Here's how the part is built. I have some questions about the finished solid (model axes, mm). A direction names the side the tool comes from. Give positions to 0.01 mm unless a question says otherwise; leave off trailing zeros. Order: outer loops, then holes, each group sorted by start corner. A loop starts at its lowest first (then second) coordinate and runs counter-clockwise, first axis right, second up.
Autodesk Inventor part; units mm, degrees
ref_plane "YZ Plane" through (0, 0, 0) normal (1, 0, 0) x (0, 1, 0)
ref_plane "XZ Plane" through (0, 0, 0) normal (0, 1, 0) x (-1, 0, 0)
ref_plane "XY Plane" through (0, 0, 0) normal (0, 0, 1) x (1, 0, 0)
sketch "Sketch1" plane through (0, 0, 0) normal (1, 0, 0) x (0, 1, 0)
  circle A0 centre (0, 0) radius 4.25
  circle A1 centre (40, 0) radius 4.25
  circle A2 centre (40, -30) radius 4.25
  circle A3 centre (0, -30) radius 4.25
  circle A4 centre (20, -60) radius 4.25
  line L0 (54.25, 0) -> (54.25, -30)
  line L1 (20, -74.25) -> (54.25, -30)
  line L2 (-14.25, -30) -> (20, -74.25)
  line L3 (-14.25, -30) -> (-14.25, 0)
  line L4 (0, 14.25) -> (54.25, 14.25)
  line L5 (54.25, 14.25) -> (-14.25, 14.25)
  line L6 (-14.25, 14.25) -> (-14.25, 0)
  line L7 (54.25, 14.25) -> (54.25, 0)
  dimension "d6" = 8.5
  dimension "d9" = 8.5
  dimension "d10" = 14.25
  dimension "d11" = 14.25
  dimension "d13" = 14.25
extrude "Extrusion1" add sketch "Sketch1" along normal blind 10
fillet "Fillet1" radius 7 5 edges at (5, 20, -74.25) (5, 54.25, -30) (5, 54.25, 14.25) (5, -14.25, 14.25) (5, -14.25, -30)
sketch "Sketch2" plane through (10, 0, 0) normal (1, 0, 0) x (0, 0, -1)
  circle A0 centre (0, 40) radius 4.25
  line L0 (0, 28) -> (30, 28)
  line L1 (0, 0) -> (0, 12)
  line L2 (0, 12) -> (30, 12)
  circle A1 centre (60, 20) radius 4.25
  arc A2 (45.061, 16.1433) -> (45.061, 23.8567) centre (44, 20) ccw
  line L3 (30, 28) -> (45.061, 23.8567)
  line L4 (30, 12) -> (45.061, 16.1433)
  line L5 (-14.25, 47.25) -> (-14.25, -7.25)
  line L6 (-2.25, 28) -> (0, 28)
  line L7 (-2.25, 28) -> (-2.25, 12)
  line L8 (-2.25, 12) -> (0, 12)
extrude "Extrusion2" cut sketch "Sketch2" against normal up to surface (10 mm away) contours L0 L3 A2 L4 L2 L8 L7 L6
fillet "Fillet2" radius 5 4 edges at (5, 12, -30) (5, 28, -30) (5, 28, 2.25) (5, 12, 2.25)
properties part number "din_motor_connector"
Q1. If we section it at D-D on y = 40: List the corners of the cut face in (x, z) for me.
Filled sheet:
outline: (0, -48.41) - (10, -48.41) - (10, -34.25) - (0, -34.25) - close; (0, -25.75) - (10, -25.75) - (10, -4.25) - (0, -4.25) - close; (0, 4.25) - (10, 4.25) - (10, 14.25) - (0, 14.25) - close
Q2. If we section it at A-A on z = -11.5: List the corners of the cut face in (x, y) for me.
Filled sheet:
outline: (0, -14.25) - (10, -14.25) - (10, 12) - (0, 12) - close; (0, 28) - (10, 28) - (10, 54.25) - (0, 54.25) - close
Q3. If we section it at C-C on y = 20: List the corners of the cut face in (x, z) for me.
Filled sheet:
outline: (0, -69.81) - (10, -69.81) - (10, -64.25) - (0, -64.25) - close; (0, -55.75) - (10, -55.75) - (10, -48) - (0, -48) - close; (0, 2.25) - (10, 2.25) - (10, 14.25) - (0, 14.25) - close
Q4. If we section it at B-B on x = 4.5: List the corners of the cut face in (y, z) for me.
Filled sheet:
outline: (-14.25, -27.61) arc R7 ccw to (-12.79, -31.89) - (14.46, -67.1) arc R7 ccw to (25.54, -67.1) - (52.79, -31.89) arc R7 ccw to (54.25, -27.61) - (54.25, 7.25) arc R7 ccw to (47.25, 14.25) - (-7.25, 14.25) arc R7 ccw to (-14.25, 7.25) - close; hole circle Ø8.5 at (0, -30); hole circle Ø8.5 at (0, 0); hole (12, -29.32) arc R5 ccw to (12.18, -30.65) - (16.14, -45.06) arc R4 ccw to (23.86, -45.06) - (27.82, -30.65) arc R5 ccw to (28, -29.32) - (28, -2.75) arc R5 ccw to (23, 2.25) - (17, 2.25) arc R5 ccw to (12, -2.75) - close; hole circle Ø8.5 at (20, -60); hole circle Ø8.5 at (40, -30); hole circle Ø8.5 at (40, 0)
Q5. I need wall thicknesses on L1, parallel to Y at x = 2.25, z = 3; L2, parallel to Z at x = 6.25, y = 40; L3, parallel to Z at x = 6, y = 20. Which ranges of each line are inside material? Lowest first, please.
Filled sheet:
L1: y = -14.25 to -3.01, 3.01 to 36.99, 43.01 to 54.25
L2: z = -48.41 to -34.25, -25.75 to -4.25, 4.25 to 14.25
L3: z = -69.81 to -64.25, -55.75 to -48, 2.25 to 14.25
Q6. For faces 4 (the face through (5, 28, -16)), 5 (the face through (5.07, 53.863, -29.902)), which set-ups out of +Z, -Z, +X, -X, +Y, -Y let a thin tool reach every point of the face, with its end or its side?
Filled sheet:
face 4: +X, -X
face 5: -Z, +X, -X, +Y
Q7. Thinking about a two-plate mould opening in Y: for faces 1 (the face through (5, -14.25, -10)), 2 (the face through (0, 4, -18)), 3 (the face through (4.93, 26.5, 0.82)), which applies, released by +Y, released by -Y, zero draft, split by the parting line, or undercut?
Filled sheet:
face 1: released by -Y
face 2: zero draft
face 3: undercut
Q8. I'm going to push flat-ended pins straight in: P1, Ø4, axis at x = 2.5, y = 14, coming from the -Z side; P2, Ø3, axis at x = 8.5, y = -5, coming from the -Z side. Where does each tip first touch, or does it pass through?
Filled sheet:
P1: stops at z = -68.56
P2: stops at z = -43.89
